Geometry check sheet. Reference: drawing and pictorial views, mm from the part's lowest x, y, z. Round coordinates to 2 decimals unless told otherwise and drop trailing zeros. Write each loop counter-clockwise with the first axis right and the second up, starting at its lowest first coordinate (ties: lowest second). Pieces come first, ordered by that corner, then holes. Notation, with made-up numbers: (-31.75, 41) - (15.25, 41) arc R30 ccw to (15.25, 80) - close; hole circle Ø3 at (77.5, 13.25). An arc over 180 degrees is marked (long way). Return JSON: item names as keys, results as strings.
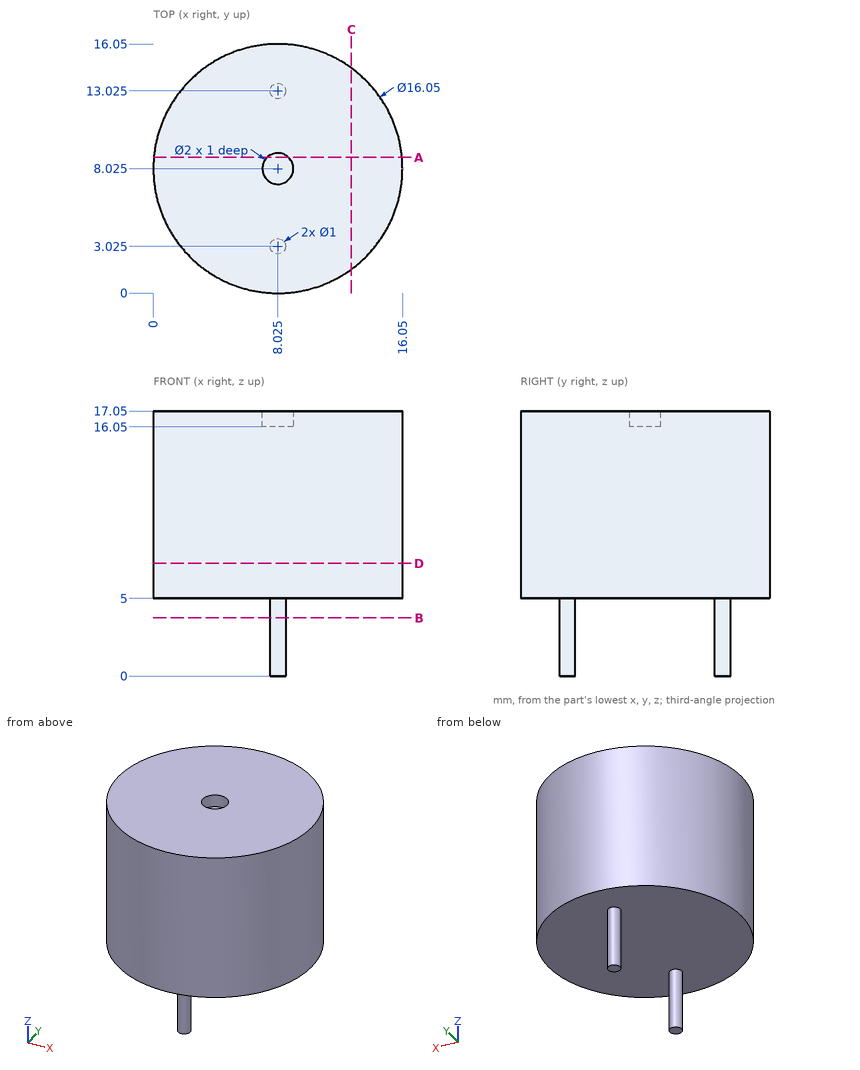
(1) Section check C-C, the plane x = 12.75. Enter the section's corners in (y, z), plus the area to 3 significant figures.
Response values:
{"outline": "(1.54, 5) - (14.51, 5) - (14.51, 17.05) - (1.54, 17.05) - close", "area": "156 mm^2"}
(2) Section check B-B, the plane z = 3.75. Enter the section's corners in (x, y) (3 decimals).
Response values:
{"outline": "circle Ø1 at (8.025, 3.025); circle Ø1 at (8.025, 13.025)"}
(3) Material ranges on line 1 along Z through (x, y) = (8, 6); line 2 along X through (y, z) = (8.5, 12); line 3 along Y through (x, z) = (7.25, 8.5), recorded low to high. Write a range as [from, to].
Response values:
{"line 1": "z = [5, 17.05]", "line 2": "x = [0.01, 16.04]", "line 3": "y = [0.04, 16.01]"}
(4) Section check A-A, the plane y = 8.75. Enter the section's corners in (x, z), plus the area to 3 significant figures.
Response values:
{"outline": "(0.03, 5) - (16.02, 5) - (16.02, 17.05) - (8.71, 17.05) - (8.71, 16.05) - (7.34, 16.05) - (7.34, 17.05) - (0.03, 17.05) - close", "area": "191 mm^2"}
(5) Section check D-D, the plane z = 7.25. Enter the section's corners in (x, y) (3 decimals).
Response values:
{"outline": "circle Ø16.05 at (8.025, 8.025)"}
(6) Gauge pin test, flat ends, axial feed: pin 1 (1 mm diameter, centred on x = 10.5, y = 7, fed in from -Z); pin 2 (5 mm diameter, centred on y = 6.5, z = 6.5, fed in from -X); pin 3 (3 mm diameter, centred on y = 3.5, z = 15, fed in from +X); pin 4 (1.5 mm diameter, centred on x = 4, z = 5, fed in from +Y). Record the tip position at first contact, or that the pin passes through.
Response values:
{"pin 1": "stops at z = 5", "pin 2": "stops at x = 0", "pin 3": "stops at x = 15.46", "pin 4": "stops at y = 15.35"}
